Geometry check sheet. Reference: the model listing, model coordinates, mm. A direction names the side the tool comes from. Round coordinates to 2 decimals unless told otherwise and drop trailing zeros. Write each loop counter-clockwise with the first axis right and the second up, starting at its lowest first coordinate (ties: lowest second). Pieces come first, ordered by that corner, then holes. Notation, with made-up numbers: (-12.75, -19) -> (41.25, -19) arc R35 cw to (41.25, 13) -> close; hole circle Ø1 at (21.25, 62). An arc over 180 degrees is marked (long way). One line per question, with ' | ' between items.
```python
from build123d import *

# Parameters (mm, degrees)
BOSS_EXTRUDE1_DEPTH = 20
SKETCH2_R           = 2.5
CUT_EXTRUDE1_DEPTH  = 6
SKETCH3_R           = 2.5
CUT_EXTRUDE2_DEPTH  = 6


with BuildPart() as part:
    # Sketch1 → Boss-Extrude1 (new body)
    with BuildSketch(Plane(origin=(0, 0, 0), x_dir=(0, 0, -1), z_dir=(1, 0, 0))):
        Polygon((0, 0), (0, 25), (5, 25), (5, 5), (25, 5), (25, 0), align=None)
    extrude(amount=BOSS_EXTRUDE1_DEPTH)

    # Sketch2 → Cut-Extrude1 (cut, through all)
    with BuildSketch(Plane(origin=(0, 5, 0), x_dir=(1, 0, 0), z_dir=(0, 1, 0))):
        with Locations((10, 15)):
            Circle(SKETCH2_R)
    extrude(amount=-CUT_EXTRUDE1_DEPTH, mode=Mode.SUBTRACT)

    # Sketch3 → Cut-Extrude2 (cut, through all)
    with BuildSketch(Plane(origin=(0, 0, -5), x_dir=(-1, 0, 0), z_dir=(0, 0, -1))):
        with Locations((-10, 15)):
            Circle(SKETCH3_R)
    extrude(amount=-CUT_EXTRUDE2_DEPTH, mode=Mode.SUBTRACT)


solid = part.part
```
(1) Sectioned sample at B-B on x = 10. Record the cut outline in (y, z).
Resolved:
outline: (0, -25) -> (5, -25) -> (5, -17.5) -> (0, -17.5) -> close; (0, -12.5) -> (5, -12.5) -> (5, -5) -> (12.5, -5) -> (12.5, 0) -> (0, 0) -> close; (17.5, -5) -> (25, -5) -> (25, 0) -> (17.5, 0) -> close
(2) Sectioned sample at C-C on y = 15. Record the cut outline in (x, z), then the cut area to 3 significant figures.
Resolved:
outline: (0, -5) -> (7.5, -5) -> (7.5, 0) -> (0, 0) -> close; (12.5, -5) -> (20, -5) -> (20, 0) -> (12.5, 0) -> close | area: 75.0 mm2
(3) Access from +Z, -Z, +X, -X, +Y, -Y to the whole of each face (thin tool, end or side, straight path). Record for faces 1 (the flat face through (0, 7, -4)), 2 (the flat face through (8, 17, -5)).
Resolved:
face 1: +Z, -Z, -X, +Y, -Y | face 2: -Z, +X, -X, +Y
(4) Go/stop test with a flat-tipped pin: pin 1 (10 mm diameter, centred on x = 6.5, y = 16, fed in from -Z). Record where the tip stops, or that it passes through.
Resolved:
pin 1: stops at z = -5
(5) Material ranges on line 1 (X direction, y = 1.25, z = -15); line 2 (Z direction, x = 18.5, y = 9); line 3 (Z direction, x = 10, y = 1.3), recorded low to high.
Resolved:
line 1: x = 0 to 7.5, 12.5 to 20 | line 2: z = -5 to 0 | line 3: z = -25 to -17.5, -12.5 to 0
(6) Sectioned sample at A-A on z = -15. Record the cut outline in (x, y).
Resolved:
outline: (0, 0) -> (7.5, 0) -> (7.5, 5) -> (0, 5) -> close; (12.5, 0) -> (20, 0) -> (20, 5) -> (12.5, 5) -> close
(7) Draft check along X on faces 3 (the flat face through (20, 7, -4)), 4 (the cylindrical face through (12, 13.5, -2.5)), 5 (the flat face through (8, 5, -13)). Enter one of: +X half, -X half, draft (parallel to the pull), parting line (faces both ways), or undercut.
Resolved:
face 3: +X half | face 4: undercut | face 5: draft
(8) Sectioned sample at D-D on y = 3.75. Record the cut outline in (x, z).
Resolved:
outline: (0, -25) -> (20, -25) -> (20, 0) -> (0, 0) -> close; hole circle Ø5 at (10, -15)
